For this review, take the finished solid that the model builds, in its own axes (mm). A direction names the side the tool comes from. Coordinates: 2 decimals unless noted, no trailing zeros. Order: outer loops, then holes, each group sorted by start corner. A loop starts at its lowest first (then second) coordinate and runs counter-clockwise, first axis right, second up.
Autodesk Fusion 360 part; units mm, degrees
sketch "Sketch1" plane through (0, 0, 0) normal (0, 0, 1) x (1, 0, 0)
  line L0 (36, 54) -> (-36, 54)
  line L1 (-36, 54) -> (-36, -54)
  line L2 (-36, -54) -> (36, -54)
  line L3 (36, -54) -> (36, 54)
  line L4 (36, 54) -> (-36, -54) construction
  line L5 (-36, 54) -> (36, -54) construction
  line L6 (37, 55) -> (-37, 55)
  line L7 (-37, 55) -> (-37, -55)
  line L8 (-37, -55) -> (37, -55)
  line L9 (37, -55) -> (37, 55)
  line L10 (37, 55) -> (-37, -55) construction
  line L11 (-37, 55) -> (37, -55) construction
  dimension "d1" = 72
  dimension "d2" = 108
  dimension "d3" = 74
  dimension "d4" = 110
extrude "Extrude1" add sketch "Sketch1" along normal blind 30
extrude "Extrude2" add sketch "Sketch1" along normal blind 2 contours L0 L1 L2 L3
1. Take a section at B-B, the plane x = 20.5. Give the boundary of the cut face in (y, z).
Answer below:
outline: (-55, 0) - (55, 0) - (55, 30) - (54, 30) - (54, 2) - (-54, 2) - (-54, 30) - (-55, 30) - close
2. The part is to be moulded in two halves that separate along X. For faces 1 (the face through (-1, 1, 0)), 2 (the face through (-37, 1, 15)), 3 (the face through (36, -1, 16)), say which applies: +X half, -X half, draft (parallel to the pull), parting line (faces both ways), or undercut.
Answer below:
face 1: draft
face 2: -X half
face 3: undercut
3. Machinability: for faces 4 (the face through (1, 55, 15)), 5 (the face through (-36, 1, 16)), which of the approach directions +Z, -Z, +X, -X, +Y, -Y give a long, thin tool a straight path to every point of the face, cutting with its end or side? Answer none if there is none.
Answer below:
face 4: +Z, -Z, +X, -X, +Y
face 5: +Z
4. Take a section at C-C, the plane y = -19. Give the boundary of the cut face in (x, z), plus the area to 3 significant figures.
Answer below:
outline: (-37, 0) - (37, 0) - (37, 30) - (36, 30) - (36, 2) - (-36, 2) - (-36, 30) - (-37, 30) - close
area: 204 mm2
5. Clearance check with flat-ended pins moving along their axes: pin 1 Ø1 at (x, y) = (5.5, -14.5) entering from +Z; pin 2 Ø3 at (x, y) = (-22, -8) entering from -Z. State where each tip first meets the part, or that it passes through.
Answer below:
pin 1: stops at z = 2
pin 2: stops at z = 0
6. Take a section at A-A, the plane z = 17. Give the boundary of the cut face in (x, y), plus the area to 3 significant figures.
Answer below:
outline: (-37, -55) - (37, -55) - (37, 55) - (-37, 55) - close; hole (-36, -54) - (36, -54) - (36, 54) - (-36, 54) - close
area: 364 mm2
7. To check wall thickness, follow L1, parallel to X at y = 13.5, z = 15.5; L2, parallel to Y at x = 6.5, z = 6; L3, parallel to Z at x = 28, y = -40. State the ranges of each line that lie inside material, in increasing order.
Answer below:
L1: x = -37 to -36, 36 to 37
L2: y = -55 to -54, 54 to 55
L3: z = 0 to 2
